The listing builds one solid part. Answer for the finished solid, in the listing's coordinates (mm). Round coordinates to 2 decimals unless told otherwise and drop trailing zeros. Write each loop counter-clockwise with the first axis right and the second up, starting at its lowest first coordinate (ties: lowest second). Pieces come first, ordered by that corner, then holes. Notation, with made-up numbers: (-7, 4.5) - (0, 4.5) arc R10 cw to (0, 13.5) - close; hole circle Ø6 at (6.25, -16). An arc over 180 degrees is marked (long way). Return JSON: item names as keys, results as strings. Group by question number.
(1) Section C-C, the plane x = 905 is taken. Write down the section's boundary in (y, z), then the cut area to 3 significant figures.
(2) Section B-B, the plane x = 908 is taken. Write down the section's boundary in (y, z), then the cut area to 3 significant figures.
(3) Each of these flat-tipped pins is pushed along its axis until it touches: pin 1 (1 mm diameter, centred on y = 567.5, z = 0.5, fed in from +X); pin 2 (4 mm diameter, centred on x = 898, y = 550, fed in from -Z); pin 3 (1 mm diameter, centred on x = 914, z = 1.5, fed in from +Y). Where does it stop, or does it pass through?
(4) Find the intervals of material crossed by line 1 along X through (y, z) = (568, 0.85); line 2 along Y through (x, z) = (914.25, 1.8); line 3 along Y through (x, z) = (907.75, 0.75), in increasing order. Write a range as [from, to].
(5) Section A-A, the plane y = 575.5 is taken. Write down the section's boundary in (x, z), then the cut area to 3 significant figures.
(6) Section D-D, the plane y = 550 is taken. Write down the section's boundary in (x, z).
```python
from build123d import *

# Parameters (mm, degrees)
MODEL_R         = 5.050911301
MODEL_W         = 4
MODEL_H         = 2
EXTRUDE_1_DEPTH = 2


with BuildPart() as part:
    # Model → 凸台-拉伸1 (new body)
    with BuildSketch(Plane.XY):
        Polygon((913.184335601, 571.907106356), (913.184335601, 563.673975647), (915.184335601, 563.673975647), (915.184335601, 553.673975647), (913.184335601, 553.673975647), (913.184335601, 543.570261409), (897.184335601, 543.570261409), (897.184335601, 553.673975647), (895.184335601, 553.673975647), (895.184335601, 563.673975647), (897.184335601, 563.673975647), (897.184335601, 571.907106356), (895.184335601, 571.907106356), (895.184335601, 581.907106356), (897.182393273, 581.907106356), (897.184335601, 591.419721737), (913.184335601, 591.419721737), (913.184335601, 581.907106356), (915.184335601, 581.907106356), (915.184335601, 571.907106356), align=None)
        with Locations((905.143744205, 556.935517453)):
            Circle(MODEL_R, mode=Mode.SUBTRACT)
        with Locations((905.143744205, 576.845149384)):
            Circle(MODEL_R, mode=Mode.SUBTRACT)
        with Locations((909.184335601, 586.518067913)):
            Rectangle(MODEL_W, MODEL_H, mode=Mode.SUBTRACT)
        with Locations((901.184335601, 586.518067913)):
            Rectangle(MODEL_W, MODEL_H, mode=Mode.SUBTRACT)
        with Locations((909.184335601, 567.518067913)):
            Rectangle(MODEL_W, MODEL_H, mode=Mode.SUBTRACT)
        with Locations((901.184335601, 567.518067913)):
            Rectangle(MODEL_W, MODEL_H, mode=Mode.SUBTRACT)
        with Locations((909.184335601, 548.518067913)):
            Rectangle(MODEL_W, MODEL_H, mode=Mode.SUBTRACT)
        with Locations((901.184335601, 548.518067913)):
            Rectangle(MODEL_W, MODEL_H, mode=Mode.SUBTRACT)
    extrude(amount=EXTRUDE_1_DEPTH)


solid = part.part
```
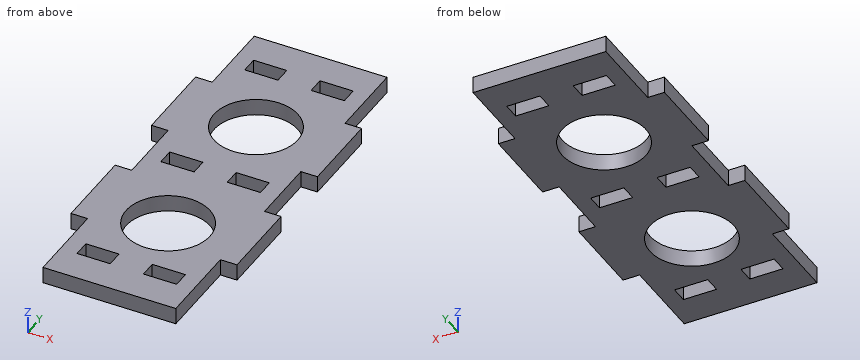
Working result:
{
 "1": {"outline": "(543.57, 0) - (551.89, 0) - (551.89, 2) - (543.57, 2) - close; (561.98, 0) - (571.8, 0) - (571.8, 2) - (561.98, 2) - close; (581.89, 0) - (591.42, 0) - (591.42, 2) - (581.89, 2) - close", "area": "55.3 mm^2"},
 "2": {"outline": "(543.57, 0) - (547.52, 0) - (547.52, 2) - (543.57, 2) - close; (549.52, 0) - (552.77, 0) - (552.77, 2) - (549.52, 2) - close; (561.1, 0) - (566.52, 0) - (566.52, 2) - (561.1, 2) - close; (568.52, 0) - (572.68, 0) - (572.68, 2) - (568.52, 2) - close; (581.01, 0) - (585.52, 0) - (585.52, 2) - (581.01, 2) - close; (587.52, 0) - (591.42, 0) - (591.42, 2) - (587.52, 2) - close", "area": "50.4 mm^2"},
 "3": {"pin 1": "stops at x = 913.18", "pin 2": "stops at z = 0", "pin 3": "stops at y = 581.91"},
 "4": {"line 1": "x = [897.18, 899.18], [903.18, 907.18], [911.18, 913.18]", "line 2": "y = [553.67, 563.67], [571.91, 581.91]", "line 3": "y = [543.57, 547.52], [549.52, 552.61], [561.26, 566.52], [568.52, 572.52], [581.17, 585.52], [587.52, 591.42]"},
 "5": {"outline": "(895.18, 0) - (900.28, 0) - (900.28, 2) - (895.18, 2) - close; (910.01, 0) - (915.18, 0) - (915.18, 2) - (910.01, 2) - close", "area": "20.5 mm^2"},
 "6": {"outline": "(897.18, 0) - (913.18, 0) - (913.18, 2) - (897.18, 2) - close"}
}
